Verification items for this drawing (mm, ordinates from the low corner). A direction names the side the tool comes from. Round coordinates to 2 decimals unless told otherwise and drop trailing zeros. Order: outer loops, then holes, each group sorted by start corner. A loop starts at its lowest first (then second) coordinate and runs counter-clockwise, first axis right, second up. Notation, with made-up numbers: (39.25, -21.75) -> (60.25, -21.75) arc R16 cw to (60.25, -3.75) -> close; hole circle Ø1 at (-40, 12.5). An arc over 180 degrees is marked (long way). Answer in a Markdown table with one row per item.
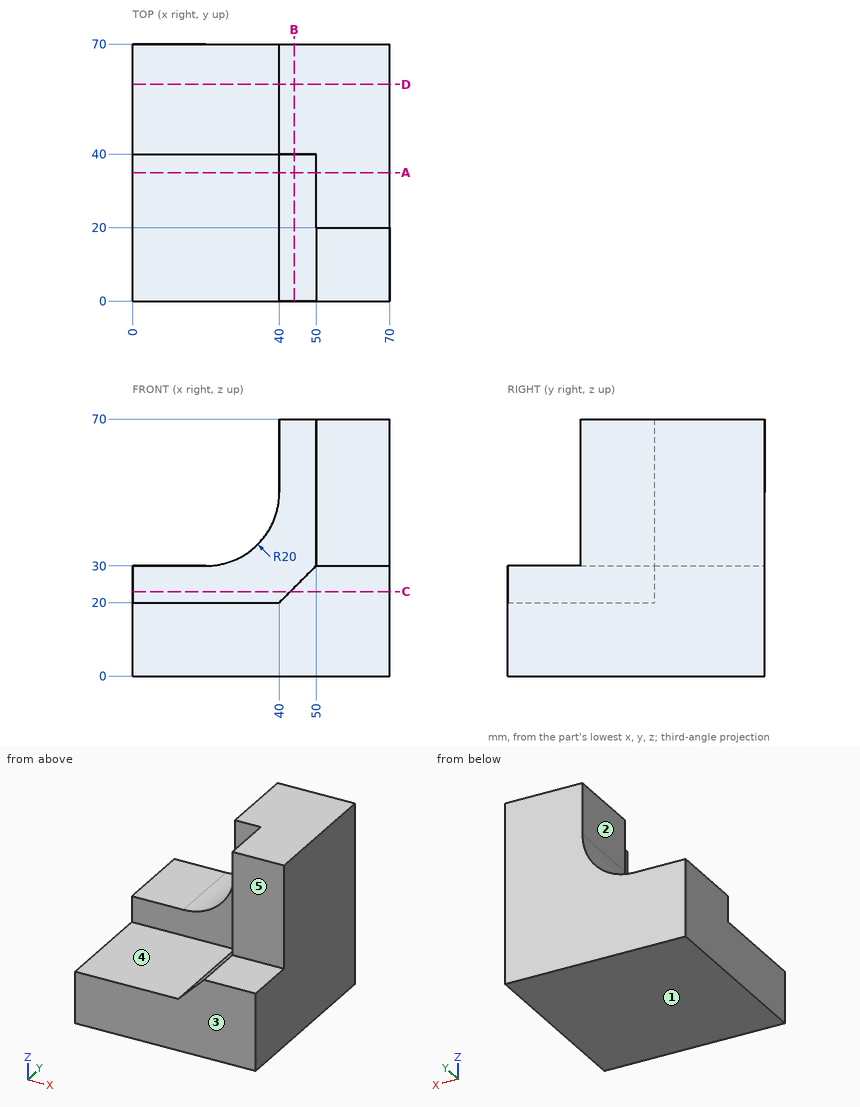
Item 1: Depth check by flat-ended pin: P1, Ø4, axis at x = 14, y = 52.5, coming from the +Z side; P2, Ø25, axis at x = 20, z = 35, coming from the -Y side; P3, Ø22, axis at y = 28.5, z = 46, coming from the -X side. Enter the tip coordinate at first touch or a pass-through.
Result sheet:
| item | result |
|---|---|
| P1 | stops at z = 30 |
| P2 | stops at y = 40 |
| P3 | stops at x = 50 |
Item 2: Cross-section at C-C (z = 23). Record the boundary of the cut face in (x, y), and give its area (3 significant figures).
Result sheet:
| item | result |
|---|---|
| outline | (0, 40) -> (43, 40) -> (43, 0) -> (70, 0) -> (70, 70) -> (0, 70) -> close |
| area | 3,180 mm^2 |
Item 3: Cross-section at A-A (y = 35). Record the boundary of the cut face in (x, z), and give its area (3 significant figures).
Result sheet:
| item | result |
|---|---|
| outline | (0, 0) -> (70, 0) -> (70, 70) -> (50, 70) -> (50, 30) -> (40, 20) -> (0, 20) -> close |
| area | 2,450 mm^2 |
Item 4: Scan lines: line 1 (Z direction, x = 40, y = 15.5); line 2 (X direction, y = 22, z = 47.5); line 3 (Z direction, x = 65, y = 17.5). Record each from-to range of solid material in increasing order. Write a range as [from, to].
Result sheet:
| item | result |
|---|---|
| line 1 | z = [0, 20] |
| line 2 | x = [50, 70] |
| line 3 | z = [0, 30] |
Item 5: Cross-section at B-B (x = 44). Record the boundary of the cut face in (y, z).
Result sheet:
| item | result |
|---|---|
| outline | (0, 0) -> (70, 0) -> (70, 70) -> (40, 70) -> (40, 24) -> (0, 24) -> close |
Item 6: Cross-section at D-D (y = 59). Record the boundary of the cut face in (x, z), and give its area (3 significant figures).
Result sheet:
| item | result |
|---|---|
| outline | (0, 0) -> (70, 0) -> (70, 70) -> (40, 70) -> (40, 50) arc R20 cw to (20, 30) -> (0, 30) -> close |
| area | 3,390 mm^2 |
Item 7: Set-up check for the marked faces 1, 2, 3, 4 and 5: record each of +Z, -Z, +X, -X, +Y, -Y from which the full face is reachable in a straight line by a thin tool's end or side.
Result sheet:
| item | result |
|---|---|
| face 1 | -Z, +X, -X, +Y, -Y |
| face 2 | +Z, -X, +Y, -Y |
| face 3 | +Z, -Z, +X, -X, -Y |
| face 4 | +Z, -X, -Y |
| face 5 | +Z, +X, -X, -Y |
